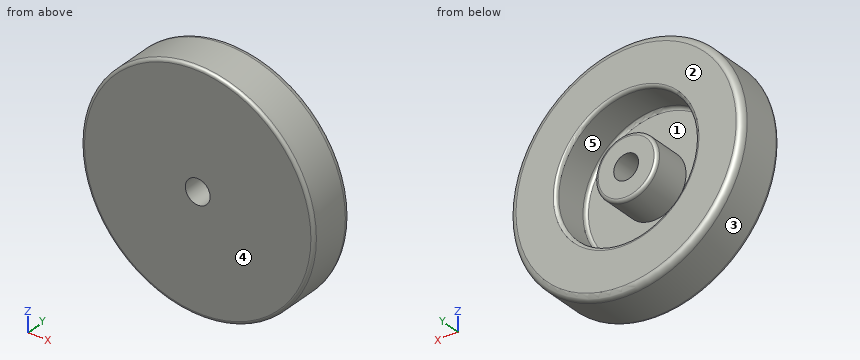
Autodesk Inventor part; units mm, degrees
ref_plane "YZ Plane" through (0, 0, 0) normal (1, 0, 0) x (0, 1, 0)
ref_plane "XZ Plane" through (0, 0, 0) normal (0, 1, 0) x (-1, 0, 0)
ref_plane "XY Plane" through (0, 0, 0) normal (0, 0, 1) x (1, 0, 0)
sketch "Esquisse1" plane through (0, 0, 0) normal (0, 1, 0) x (-1, 0, 0)
  circle A0 centre (0, 0) radius 37.5
  dimension "d0" = 75
extrude "Extrusion1" add sketch "Esquisse1" along normal blind 3
sketch "Esquisse2" plane through (0, 3, 0) normal (0, 1, 0) x (1, 0, 0)
  circle A0 centre (0, 0) radius 37.5
  circle A1 centre (0, 0) radius 10
  circle A2 centre (0, 0) radius 22.5
  dimension "d3" = 15
  dimension "d4" = 20
extrude "Extrusion2" add sketch "Esquisse2" along normal blind 12
sketch "Esquisse3" plane through (0, 15, 0) normal (0, 1, 0) x (1, 0, 0)
  circle A0 centre (0, 0) radius 10
  circle A1 centre (0, 0) radius 4
  dimension "d7" = 8
extrude "Extrusion3" cut sketch "Esquisse3" against normal through all contours A1
fillet "Congé1" radius 2 1 edges at (-37.5, 15, 0)
fillet "Congé2" radius 1 1 edges at (-10, 15, 0)
fillet "Congé3" radius 1 1 edges at (-22.5, 15, 0)
fillet "Congé4" radius 1 1 edges at (-22.5, 3, 0)
fillet "Congé5" radius 1 1 edges at (37.5, 0, 0)
properties part number "wheel"
For this review, take the finished solid that the model builds, in its own axes (mm). Face numbers are marked on the shaded views. A direction names the side the tool comes from. Give positions to 0.01 mm unless a question says otherwise; leave off trailing zeros. Write each loop counter-clockwise with the first axis right and the second up, starting at its lowest first coordinate (ties: lowest second). Pieces come first, ordered by that corner, then holes.
Item 1: Machinability: for the marked faces 1 and 2, which of the approach directions +Z, -Z, +X, -X, +Y, -Y give a long, thin tool a straight path to every point of the face, cutting with its end or side? Answer none if there is none.
Item 2: The part is to be moulded in two halves that separate along X. For the marked faces 3, 4 and 5, say which applies: +X half, -X half, draft (parallel to the pull), parting line (faces both ways), or undercut.
Item 3: Wall thickness on probe 1 along X at (y, z) = (6.5, 0); probe 2 along Z at (x, y) = (8, 12.75): over which ranges is each line inside the solid? List them lowest first.
Item 4: Take a section at A-A (y = 5.25). Give the boundary of the cut face in (x, z), and give its area (3 significant figures).
Item 5: Insertion check: P1, Ø8, axis at x = 28, y = 5, coming from the -Z side; P2, Ø1, axis at x = -18, z = 9.5, coming from the +Y side; P3, Ø3, axis at x = -13.5, y = 13, coming from the +Z side. Each pin has a flat end and moves straight along its axis. Give the tip position at first contact, or say it passes through.
Established:
1. face 1: +Y
1. face 2: +Z, -Z, +X, -X, +Y
2. face 3: parting line
2. face 4: draft
2. face 5: undercut
3. probe 1: x = -37.5 to -22.5, -10 to -4, 4 to 10, 22.5 to 37.5
3. probe 2: z = -36.64 to -21.03, -6 to 6, 21.03 to 36.64
4. outline: circle Ø75 at (0, 0); circle Ø20 at (0, 0); hole circle Ø45 at (0, 0); hole circle Ø8 at (0, 0)
4. area: 3,090 mm2
5. P1: stops at z = -28.81
5. P2: stops at y = 3
5. P3: stops at z = 35.53
